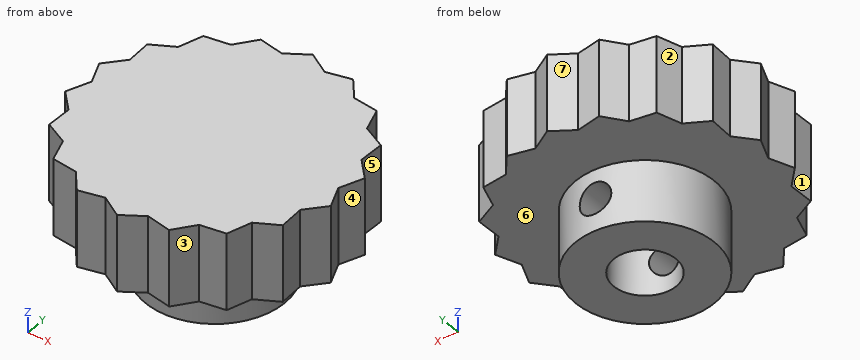
```python
from build123d import *

# Parameters (mm, degrees)
CROQUIS1_R                 = 17.5
SALIENTE_EXTRUIR1_DEPTH    = 10
CROQUIS2_R                 = 9.075
CROQUIS2_R_2               = 4.075
SALIENTE_EXTRUIR2_DEPTH    = 8
CORTAR_EXTRUIR1_START      = -10
CROQUIS3_R                 = 19
CORTAR_EXTRUIR1_DEPTH      = 10
CORTAR_EXTRUIR2_DEPTH      = 27.519152184
CORTAR_EXTRUIR2_DEPTH_BACK = 27.519152184
CROQUIS4_R                 = 2.05
CORTAR_EXTRUIR3_START      = -5
CROQUIS5_R                 = 4.075
CORTAR_EXTRUIR3_DEPTH      = 5


with BuildPart() as part:
    # Croquis1 → Saliente-Extruir1 (new body)
    with BuildSketch(Plane.XY):
        Circle(CROQUIS1_R)
    extrude(amount=SALIENTE_EXTRUIR1_DEPTH)

    # Croquis2 → Saliente-Extruir2 (add)
    with BuildSketch(Plane(origin=(0, 0, 0), x_dir=(-1, 0, 0), z_dir=(0, 0, -1))):
        with Locations(Location((0, 0, 0), (0, 0, 180))):
            Circle(CROQUIS2_R)
        Circle(CROQUIS2_R_2, mode=Mode.SUBTRACT)
    extrude(amount=SALIENTE_EXTRUIR2_DEPTH)

    # Croquis3 → Cortar-Extruir1 (cut)
    with BuildSketch(Plane.XY.offset(10).offset(CORTAR_EXTRUIR1_START)):
        Circle(CROQUIS3_R)
        Polygon((0, 17.5), (2.778370843, 15.756924048), (5.985352508, 16.444620864), (8, 13.856406461), (11.24878317, 13.405777755), (12.25671109, 10.284601755), (15.155444566, 8.75), (15.035081933, 5.472322293), (17.234135678, 3.038843109), (16, 0), (17.234135678, -3.038843109), (15.035081933, -5.472322293), (15.155444566, -8.75), (12.25671109, -10.284601755), (11.24878317, -13.405777755), (8, -13.856406461), (5.985352508, -16.444620864), (2.778370843, -15.756924048), (0, -17.5), (-2.778370843, -15.756924048), (-5.985352508, -16.444620864), (-8, -13.856406461), (-11.24878317, -13.405777755), (-12.25671109, -10.284601755), (-15.155444566, -8.75), (-15.035081933, -5.472322293), (-17.234135678, -3.038843109), (-16, 0), (-17.234135678, 3.038843109), (-15.035081933, 5.472322293), (-15.155444566, 8.75), (-12.25671109, 10.284601755), (-11.24878317, 13.405777755), (-8, 13.856406461), (-5.985352508, 16.444620864), (-2.778370843, 15.756924048), align=None, mode=Mode.SUBTRACT)
    extrude(amount=CORTAR_EXTRUIR1_DEPTH, mode=Mode.SUBTRACT)

    # Croquis4 → Cortar-Extruir2 (cut, two sides: drawn at the far end of the back side and taken through both)
    with BuildSketch(Plane(origin=(0, 0, 0), x_dir=(1, 0, 0), z_dir=(0, 1, 0)).offset(-CORTAR_EXTRUIR2_DEPTH_BACK)):
        with Locations(Location((0, 3.75, 0), (0, 0, 270))):
            Circle(CROQUIS4_R)
    extrude(amount=CORTAR_EXTRUIR2_DEPTH + CORTAR_EXTRUIR2_DEPTH_BACK, mode=Mode.SUBTRACT)

    # Croquis5 → Cortar-Extruir3 (cut)
    with BuildSketch(Plane(origin=(0, 0, 0), x_dir=(-1, 0, 0), z_dir=(0, 0, -1)).offset(CORTAR_EXTRUIR3_START)):
        Circle(CROQUIS5_R)
    extrude(amount=CORTAR_EXTRUIR3_DEPTH, mode=Mode.SUBTRACT)


solid = part.part
```
Geometry: final body of the model. Coordinates: model frame, mm. Face numbers are marked on the shaded views. A direction names the side the tool comes from. Round coordinates to 2 decimals unless told otherwise and drop trailing zeros. Loops run counter-clockwise (first coordinate to the right, second up) from the corner with the lowest first, then second, coordinate; pieces in that order, holes last.
Item 1: Contact query for flat-ended pins moving along their axis: P1, Ø3, axis at y = -10, z = 6.5, coming from the -X side; P2, Ø5, axis at x = -1.5, z = -1.5, coming from the -Y side; P3, Ø6, axis at y = 2.5, z = -3.5, coming from the +X side (3 decimals); P4, Ø5.5, axis at x = 0, z = -3.75, coming from the +Y side (3 decimals). Output: stop coordinate, or through.
Checked values:
P1: stops at x = -15.16
P2: stops at y = -17.5
P3: stops at x = 9.075
P4: stops at y = 9.075
Item 2: Section A-A, the plane z = -0.5. Output: boundary loops of the cut face in (x, y) (3 decimals).
Checked values:
outline: circle Ø18.15 at (0, 0); hole circle Ø8.15 at (0, 0)
Item 3: Section C-C, the plane z = -3.75. Output: boundary loops of the cut face in (x, y) (3 decimals), plus the area to 3 significant figures.
Checked values:
outline: (-2.05, -8.84) - (-2.05, -3.522) arc R4.075 cw to (-2.05, 3.522) - (-2.05, 8.84) arc R9.075 ccw to start; (2.05, -8.84) arc R9.075 ccw to (2.05, 8.84) - (2.05, 3.522) arc R4.075 cw to (2.05, -3.522) - close
area: 165 mm2
Item 4: Section D-D, the plane x = -13.5. Output: boundary loops of the cut face in (y, z).
Checked values:
outline: (-9.63, 0) - (9.63, 0) - (9.63, 10) - (-9.63, 10) - close
Item 5: Line query: L1, parallel to Z at x = 0, y = 7.1; L2, parallel to Y at x = 0, z = 1.25 (3 decimals); L3, parallel to X at y = -7.9, z = -3.75. Output: solid intervals per line, ascending.
Checked values:
L1: z = -8 to -5.8, -1.7 to 10
L2: y = -17.5 to -4.075, 4.075 to 17.5
L3: x = -4.47 to -2.05, 2.05 to 4.47
Item 6: Reachability of the marked faces 5, 6 and 7 from +Z, -Z, +X, -X, +Y, -Y: full face, straight path, thin tool, end or side. Return the list, or none.
Checked values:
face 5: +Z, -Z, +X
face 6: -Z
face 7: +Z, -Z, +Y
Item 7: Mould query, pull axis Y, two halves, no side actions, for the marked faces 1, 2, 3 and 4. Classes: released by +Y, released by -Y, zero draft, split by the parting line, or undercut.
Checked values:
face 1: undercut
face 2: released by +Y
face 3: released by -Y
face 4: undercut
Item 8: Section B-B, the plane y = -2.5. Output: boundary loops of the cut face in (x, z), plus the area to 3 significant figures.
Checked values:
outline: (-17.02, 0) - (-8.72, 0) - (-8.72, -8) - (-3.22, -8) - (-3.22, 5) - (3.22, 5) - (3.22, -8) - (8.72, -8) - (8.72, 0) - (17.02, 0) - (17.02, 10) - (-17.02, 10) - close
area: 396 mm2
